Here's how the part is built. I have some questions about the finished solid (model axes, mm). Face numbers are marked on the shaded views. Round coordinates to 2 decimals unless told otherwise and drop trailing zeros. Order: outer loops, then holes, each group sorted by start corner. A loop starts at its lowest first (then second) coordinate and runs counter-clockwise, first axis right, second up. Notation, with made-up numbers: (18, 50.25) - (66, 50.25) arc R13 cw to (66, 67.25) - close; hole circle Ø11 at (4.5, 62). An arc over 180 degrees is marked (long way). One line per item, written item: value.
from build123d import *

# Parameters (mm, degrees)
F0_W     = 66.04
F0_H     = 40.64
F1_DEPTH = 35.56
F2_R     = 5.08
F3_T     = -2.54


with BuildPart() as f1:
    # F0 (on Front) → F1 (new body)
    with BuildSketch(Plane.XZ):
        Rectangle(F0_W, F0_H)
    extrude(amount=F1_DEPTH)

    # F2
    f2_edges = [f1.edges().sort_by_distance(p)[0] for p in [
        (33.02, -35.56, 0),
        (33.02, 0, 0),
        (-33.02, -35.56, 0),
        (-33.02, 0, 0),
    ]]
    fillet(f2_edges, radius=F2_R)

    # F3
    f3_openings = [f1.faces().sort_by_distance(p)[0] for p in [
        (0, -17.78, 20.32),
    ]]
    offset(amount=F3_T, openings=f3_openings)


solid = f1.part
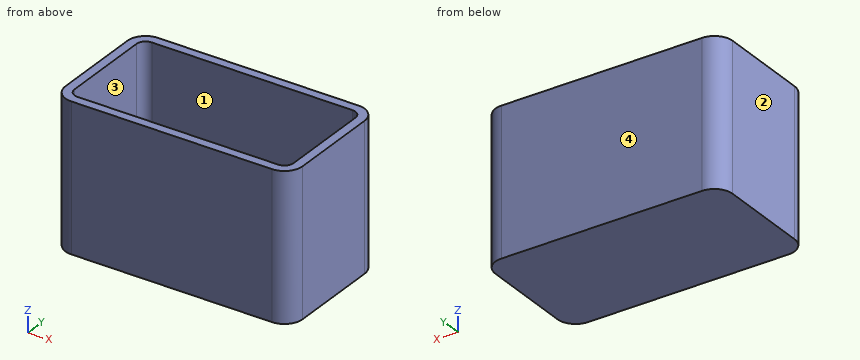
Q1. If we section it at B-B, the plane x = 0.5: Please give me the cut outline in (y, z).
Results list:
outline: (-35.56, -20.32) - (0, -20.32) - (0, 20.32) - (-2.54, 20.32) - (-2.54, -17.78) - (-33.02, -17.78) - (-33.02, 20.32) - (-35.56, 20.32) - close
Q2. If I drill on line 1 along X through (y, z) = (-25, -5.5); line 2 along Y through (x, z) = (19.5, 19.5); line 3 along Z through (x, y) = (-26, -27), over which ranges is the centre line in solid material (lowest first)?
Results list:
line 1: -33.02 to -30.48, 30.48 to 33.02
line 2: -35.56 to -33.02, -2.54 to 0
line 3: -20.32 to -17.78
Q3. Will this pin go through, and if not, where does the flat tip stop? pin 1 (9 mm diameter, centred on x = -13.5, y = -16.5, fed in from +Z).
Results list:
pin 1: z = -17.78
Q4. We'd pull the mould along X, two halves only. Please class the marked faces 1, 2, 3 and 4: released by +X, released by -X, zero draft, split by the parting line, or undercut.
Results list:
face 1: undercut
face 2: released by -X
face 3: undercut
face 4: zero draft
Q5. If we section it at A-A, the plane z = -5: Please give me the cut outline in (x, y).
Results list:
outline: (-33.02, -30.48) arc R5.08 ccw to (-27.94, -35.56) - (27.94, -35.56) arc R5.08 ccw to (33.02, -30.48) - (33.02, -5.08) arc R5.08 ccw to (27.94, 0) - (-27.94, 0) arc R5.08 ccw to (-33.02, -5.08) - close; hole (-30.48, -30.48) arc R2.54 ccw to (-27.94, -33.02) - (27.94, -33.02) arc R2.54 ccw to (30.48, -30.48) - (30.48, -5.08) arc R2.54 ccw to (27.94, -2.54) - (-27.94, -2.54) arc R2.54 ccw to (-30.48, -5.08) - close
Q6. If we section it at C-C, the plane y = -16.5: Please give me the cut outline in (x, z).
Results list:
outline: (-33.02, -20.32) - (33.02, -20.32) - (33.02, 20.32) - (30.48, 20.32) - (30.48, -17.78) - (-30.48, -17.78) - (-30.48, 20.32) - (-33.02, 20.32) - close
